```python
from build123d import *

# Parameters (mm, degrees)
BOSS_EXTRUDE1_DEPTH = 20
CUT_EXTRUDE1_DEPTH  = 28.202941017
CUT_EXTRUDE2_DEPTH  = 10
CUT_EXTRUDE3_DEPTH  = 10
SKETCH5_W           = 8
SKETCH5_H           = 10
CUT_EXTRUDE4_DEPTH  = 2


with BuildPart() as part:
    # Sketch1 → Boss-Extrude1 (new body)
    with BuildSketch(Plane(origin=(0, 0, 0), x_dir=(1, 0, 0), z_dir=(0, 1, 0))):
        with BuildLine():
            Line((-7, -12), (-7, 0))
            ThreePointArc((-7, 0), (0, 7), (7, 0))
            Line((7, 0), (7, -12))
            Line((7, -12), (1, -12))
            Line((1, -12), (1, -3.872983346))
            ThreePointArc((1, -3.872983346), (0, 4), (-1, -3.872983346))
            Line((-1, -3.872983346), (-1, -12))
            Line((-1, -12), (-7, -12))
        make_face()
    extrude(amount=BOSS_EXTRUDE1_DEPTH)

    # Sketch2 → Cut-Extrude1 (cut, through all)
    with BuildSketch(Plane.ZY.offset(7)):
        with BuildLine():
            Line((6.409009742, 6.590990258), (8, 8.181980515))
            Line((8, 8.181980515), (9.590990258, 6.590990258))
            ThreePointArc((9.590990258, 6.590990258), (8, 2.75), (6.409009742, 6.590990258))
        make_face()
    extrude(amount=-CUT_EXTRUDE1_DEPTH, mode=Mode.SUBTRACT)

    # Sketch3 → Cut-Extrude2 (cut)
    with BuildSketch(Plane(origin=(0, 20, 0), x_dir=(1, 0, 0), z_dir=(0, 1, 0))):
        Polygon((1, -4), (-7, -4), (-7, 7), (7, 7), (7, 0), (7, -12), (1, -12), align=None)
    extrude(amount=-CUT_EXTRUDE2_DEPTH, mode=Mode.SUBTRACT)

    # Sketch4 → Cut-Extrude3 (cut)
    with BuildSketch(Plane(origin=(-1, 0, 0), x_dir=(0, 0, -1), z_dir=(1, 0, 0))):
        with BuildLine():
            Line((-9.237436867, 16.237436867), (-8, 17.474873734))
            Line((-8, 17.474873734), (-6.762563133, 16.237436867))
            ThreePointArc((-6.762563133, 16.237436867), (-8, 13.25), (-9.237436867, 16.237436867))
        make_face()
    extrude(amount=-CUT_EXTRUDE3_DEPTH, mode=Mode.SUBTRACT)

    # Sketch5 → Cut-Extrude4 (cut)
    with BuildSketch(Plane.ZY.offset(7)):
        with Locations((8, 15)):
            Rectangle(SKETCH5_W, SKETCH5_H)
    extrude(amount=-CUT_EXTRUDE4_DEPTH, mode=Mode.SUBTRACT)


solid = part.part
```
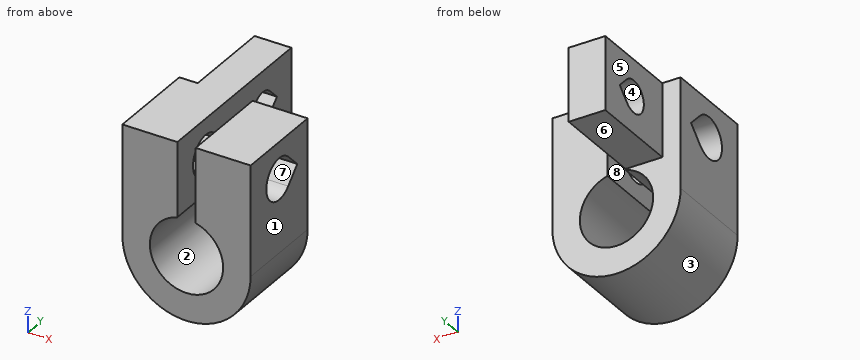
Source: CAD feature listing. Evaluate the final solid. Frame: model axes, mm. Face numbers are marked on the shaded views. A direction names the side the tool comes from. Coordinates: 2 decimals unless noted, no trailing zeros. Write each loop counter-clockwise with the first axis right and the second up, starting at its lowest first coordinate (ties: lowest second). Pieces come first, ordered by that corner, then holes. Notation, with made-up numbers: (-8, -2) -> (11, -2) arc R29 cw to (11, 27) -> close; hole circle Ø9 at (33.25, 33). An arc over 180 degrees is marked (long way). Return JSON: item names as keys, results as strings. Group by question number.
1) Mould query, pull axis X, two halves, no side actions, for the marked faces 1, 2, 3 and 4. Classes: +X half, -X half, draft (parallel to the pull), parting line (faces both ways), or undercut.
2) Contact query for flat-ended pins moving along their axis: P1, Ø3, axis at x = -2, y = 17, coming from the -Z side; P2, Ø5.5, axis at y = 15, z = 8, coming from the +X side; P3, Ø4, axis at x = 4.5, y = 9.5, coming from the -Z side. Output: stop coordinate, or through.
3) Section query D-D, the plane z = 4.25. Return loops of the section in (x, y).
4) Set-up query: the marked faces 5, 6, 7 and 8. Return all of +Z, -Z, +X, -X, +Y, -Y with unobstructed straight access to the full face (end or side cutting, diameter ignored); none if empty.
5) Section query B-B, the plane y = 15. Return loops of the section in (x, z), plus the area to 3 significant figures.
6) Section query A-A, the plane y = 5. Return loops of the section in (x, z).
7) Section query C-C, the plane x = 2. Return loops of the section in (y, z).
8) Ray query, line 1 along Y through (x, z) = (-5.5, 3.5); line 2 along Z through (x, y) = (6, 5); line 3 along X through (y, z) = (5.5, 5). Return the intervals inside material, ascending.
From the geometry:
{
 "1": {"face 1": "+X half", "face 2": "undercut", "face 3": "parting line", "face 4": "draft"},
 "2": {"P1": "z = 4", "P2": "x = -1", "P3": "z = -6.54"},
 "3": {"outline": "(-7, 0) -> (-1, 0) -> (-1, 20) -> (-5, 20) -> (-5, 10) -> (-7, 10) -> close; (1, 0) -> (7, 0) -> (7, 10) -> (1, 10) -> close"},
 "4": {"face 5": "+Z, -Z, -X, +Y", "face 6": "-Z, +X, -X, +Y", "face 7": "+X, -X", "face 8": "+Z, +Y, -Y"},
 "5": {"outline": "(-5, 4) -> (-1, 4) -> (-1, 6.25) -> (-5, 6.25) -> close; (-5, 9.75) -> (-1, 9.75) -> (-1, 12) -> (-5, 12) -> close", "area": "18.0 mm²"},
 "6": {"outline": "(-7, 0) arc R7 ccw to (7, 0) -> (7, 5.75) -> (1, 5.75) -> (1, 3.87) arc R4 cw (long way) to (-1, 3.87) -> (-1, 5.75) -> (-7, 5.75) -> close; (-7, 10.25) -> (-1, 10.25) -> (-1, 12) -> (-7, 12) -> close; (1, 10.25) -> (7, 10.25) -> (7, 12) -> (1, 12) -> close"},
 "7": {"outline": "(0, -6.71) -> (10, -6.71) -> (10, -3.46) -> (0, -3.46) -> close; (0, 3.46) -> (10, 3.46) -> (10, 12) -> (0, 12) -> close; hole (6.59, 6.41) -> (8.18, 8) -> (6.59, 9.59) arc R2.25 ccw (long way) to start"},
 "8": {"line 1": "0 to 10", "line 2": "-3.61 to 5.75, 10.25 to 12", "line 3": "-7 to -1, 1 to 7"}
}
